```python
from build123d import *

# Parameters (mm, degrees)
SKETCH_1_R      = 3.4
SKETCH_1_W      = 5
SKETCH_1_H      = 5
EXTRUDE_1_DEPTH = 205


with BuildPart() as part:
    # 草图1 → 凸台-拉伸1 (new body)
    with BuildSketch(Plane(origin=(0, 0, 0), x_dir=(0, 0, -1), z_dir=(1, 0, 0))):
        Polygon((0, 6), (4.585786438, 6), (10.718811909, 12.133025471), (11, 13), (11, 18), (5.1, 18), (5.1, 20), (20, 20), (20, 5.1), (18, 5.1), (18, 11), (13, 11), (12.133025471, 10.718811909), (6, 4.585786438), (6, 0), (6, -4.585786438), (12.133025471, -10.718811909), (13, -11), (18, -11), (18, -5.1), (20, -5.1), (20, -20), (5.1, -20), (5.1, -18), (11, -18), (11, -13), (10.718811909, -12.133025471), (4.585786438, -6), (0, -6), (-4.585786438, -6), (-10.718811909, -12.133025471), (-11, -13), (-11, -18), (-5.1, -18), (-5.1, -20), (-20, -20), (-20, -5.1), (-18, -5.1), (-18, -11), (-13, -11), (-12.133025471, -10.718811909), (-6, -4.585786438), (-6, 0), (-6, 4.585786438), (-12.133025471, 10.718811909), (-13, 11), (-18, 11), (-18, 5.1), (-20, 5.1), (-20, 20), (-5.1, 20), (-5.1, 18), (-11, 18), (-11, 13), (-10.718811909, 12.133025471), (-4.585786438, 6), align=None)
        with Locations(Location((0, 0, 0), (0, 0, 180))):
            Circle(SKETCH_1_R, mode=Mode.SUBTRACT)
        with Locations((15.5, -15.5)):
            Rectangle(SKETCH_1_W, SKETCH_1_H, mode=Mode.SUBTRACT)
        with Locations((15.5, 15.5)):
            Rectangle(SKETCH_1_W, SKETCH_1_H, mode=Mode.SUBTRACT)
        with Locations((-15.5, -15.5)):
            Rectangle(SKETCH_1_W, SKETCH_1_H, mode=Mode.SUBTRACT)
        with Locations((-15.5, 15.5)):
            Rectangle(SKETCH_1_W, SKETCH_1_H, mode=Mode.SUBTRACT)
    extrude(amount=EXTRUDE_1_DEPTH)


solid = part.part
```
Verification items for the finished model (mm, model axes). A direction names the side the tool comes from. Give positions to 0.01 mm unless a question says otherwise; leave off trailing zeros. Loops run counter-clockwise (first coordinate to the right, second up) from the corner with the lowest first, then second, coordinate; pieces in that order, holes last. Notation, with made-up numbers: M 6,69 L 28,69 A14 ccw 28,78 Z; hole C -23,-1.75 d2. An arc over 180 degrees is marked long. Return JSON: item names as keys, results as strings.
1) Tool access check on faces 4 (the flat face through (0, -3, 3)), 5 (the flat face through (101, 18, 8)). Record the directions out of +Z, -Z, +X, -X, +Y, -Y that give a thin tool (end or side, any length) a straight path to the whole face; none if there is none.
Findings:
{"face 4": "+Z, -Z, -X, +Y, -Y", "face 5": "+X, -X"}
2) Gauge pin test, flat end, axial feed: P1, Ø3, axis at x = 52, z = 0, coming from the -Y side. Record the tip position at first contact, or that the pin passes through.
Findings:
{"P1": "stops at y = -6"}
3) Section check B-B, the plane y = 16. Enter the section's corners in (x, z), and give its area (3 significant figures).
Findings:
{"outline": "M 0,-20 L 205,-20 L 205,-18 L 0,-18 Z; M 0,-13 L 205,-13 L 205,-11 L 0,-11 Z; M 0,11 L 205,11 L 205,13 L 0,13 Z; M 0,18 L 205,18 L 205,20 L 0,20 Z", "area": "1,640 mm2"}
4) Section check A-A, the plane z = 0. Enter the section's corners in (x, y), and give its area (3 significant figures).
Findings:
{"outline": "M 0,-6 L 205,-6 L 205,-3.4 L 0,-3.4 Z; M 0,3.4 L 205,3.4 L 205,6 L 0,6 Z", "area": "1,070 mm2"}
5) Mould release check, pull along Z, two halves, no side actions. Record for faces 1 (the flat face through (101, 20, -12)), 2 (the flat face through (101, -13, 20)), 3 (the flat face through (101, -16, 13)): released by +Z, released by -Z, zero draft, split by the parting line, or undercut.
Findings:
{"face 1": "zero draft", "face 2": "released by +Z", "face 3": "undercut"}
6) Section check D-D, the plane z = -9. Enter the section's corners in (x, y), and give its area (3 significant figures).
Findings:
{"outline": "M 0,-20 L 205,-20 L 205,-18 L 0,-18 Z; M 0,-10.41 L 205,-10.41 L 205,-7.59 L 0,-7.59 Z; M 0,7.59 L 205,7.59 L 205,10.41 L 0,10.41 Z; M 0,18 L 205,18 L 205,20 L 0,20 Z", "area": "1,980 mm2"}
7) Material ranges on L1, parallel to Y at x = 9, z = 17; L2, parallel to Y at x = 52, z = 0, recorded low to high. Write a range as [from, to].
Findings:
{"L1": "y = [-20, -18], [-13, -11], [11, 13], [18, 20]", "L2": "y = [-6, -3.4], [3.4, 6]"}
